```python
from build123d import *

# Parameters (mm, degrees)
SKETCH1_R           = 1.75
BOSS_EXTRUDE1_DEPTH = 3
FILLET1_R           = 0.5


with BuildPart() as part:
    # Sketch1 → Boss-Extrude1 (new body)
    with BuildSketch(Plane.XY):
        with BuildLine():
            Line((-266.5, 139.6), (-179.5, 139.6))
            Line((-179.5, 139.6), (-179.5, 127.873863542))
            ThreePointArc((-179.5, 127.873863542), (-178.955663943, 125.60515051), (-177.441176471, 123.8304144))
            ThreePointArc((-177.441176471, 123.8304144), (-176, 121), (-177.441176471, 118.1695856))
            ThreePointArc((-177.441176471, 118.1695856), (-178.955663943, 116.39484949), (-179.5, 114.126136458))
            Line((-179.5, 114.126136458), (-179.5, 102.4))
            Line((-179.5, 102.4), (-266.5, 102.4))
            Line((-266.5, 102.4), (-266.5, 110))
            Line((-266.5, 110), (-194.5, 110))
            Line((-194.5, 110), (-194.5, 134))
            Line((-194.5, 134), (-266.5, 134))
            Line((-266.5, 134), (-266.5, 139.6))
        make_face()
        with Locations((-179.5, 121)):
            Circle(SKETCH1_R, mode=Mode.SUBTRACT)
    extrude(amount=BOSS_EXTRUDE1_DEPTH)

    # Fillet1
    fillet1_edges = [part.edges().sort_by_distance(p)[0] for p in [
        (-178.955663943, 116.39484949, 0),
        (-179.5, 108.263068229, 0),
        (-179.5, 133.736931771, 3),
        (-223, 102.4, 0),
        (-266.5, 106.2, 0),
        (-230.5, 110, 0),
        (-194.5, 122, 0),
        (-230.5, 134, 0),
        (-266.5, 136.8, 0),
        (-223, 139.6, 0),
        (-179.5, 133.736931771, 0),
        (-178.955663943, 125.60515051, 0),
        (-176, 121, 0),
        (-223, 139.6, 3),
        (-266.5, 136.8, 3),
        (-230.5, 134, 3),
        (-194.5, 122, 3),
        (-181.25, 121, 0),
        (-181.25, 121, 3),
        (-230.5, 110, 3),
        (-266.5, 106.2, 3),
        (-223, 102.4, 3),
        (-179.5, 108.263068229, 3),
        (-178.955663943, 116.39484949, 3),
        (-176, 121, 3),
        (-178.955663943, 125.60515051, 3),
    ]]
    fillet(fillet1_edges, radius=FILLET1_R)


solid = part.part
```
Work out the finished part from the listing and answer in its coordinate system (mm). A direction names the side the tool comes from. Round coordinates to 2 decimals unless told otherwise and drop trailing zeros. Write each loop counter-clockwise with the first axis right and the second up, starting at its lowest first coordinate (ties: lowest second). Pieces come first, ordered by that corner, then holes. Notation, with made-up numbers: (30.5, 1) - (51.5, 1) arc R24 ccw to (51.5, 27) - close; hole circle Ø1 at (47.5, 8.25). An arc over 180 degrees is marked (long way). Return JSON: item names as keys, results as strings. Group by question number.
Q1. The part is cut by section D-D on y = 137. Write down the section's boundary in (x, z), then the cut area to 3 significant figures.
Q2. The part is cut by section B-B on z = 1.2. Write down the section's boundary in (x, y), then the cut area to 3 significant figures.
Q3. The mould has two halves that part along Y. Classify faces 5 (the cylindrical face through (-178.97, 125.63, 1.49)), 6 (the flat face through (-231, 110, 1)), 7 (the flat face through (-211, 109, 3)): released by +Y, released by -Y, zero draft, split by the parting line, or undercut.
Q4. Find the intervals of material crossed by L1, parallel to Y at x = -253.5, z = 0.5; L2, parallel to X at y = 121, z = 1.2; L3, parallel to X at y = 105, z = 1.2, in increasing order.
Q5. Each of these flat-tipped pins is pushed along its axis until it touches: pin 1 Ø1.6 at (y, z) = (118.5, 1) entering from -X; pin 2 Ø12 at (x, y) = (-230, 127) entering from +Z; pin 3 Ø1.6 at (y, z) = (133.5, 1) entering from +X. Where does it stop, or does it pass through?
Q6. The part is cut by section C-C on x = -250. Write down the section's boundary in (y, z), then the cut area to 3 significant figures.
Q7. For faces 1 (the flat face through (-222, 102.4, 1)), 2 (the flat face through (-179.5, 108, 1)), 3 (the flat face through (-194.5, 122, 1)), 4 (the flat face through (-179.5, 134, 1)), determine the directions among +Z, -Z, +X, -X, +Y, -Y from which every point of the face is accessible in a straight line to the end or side of a thin tool.
Q8. The part is cut by section A-A on y = 121. Write down the section's boundary in (x, z), then the cut area to 3 significant figures.
Solved:
{
 "1": {"outline": "(-266.5, 0.5) arc R0.5 ccw to (-266, 0) - (-180, 0) arc R0.5 ccw to (-179.5, 0.5) - (-179.5, 2.5) arc R0.5 ccw to (-180, 3) - (-266, 3) arc R0.5 ccw to (-266.5, 2.5) - close", "area": "261 mm²"},
 "2": {"outline": "(-266.5, 102.4) - (-179.5, 102.4) - (-179.5, 114.13) arc R5 cw to (-177.44, 118.17) arc R3.5 ccw to (-177.44, 123.83) arc R5 cw to (-179.5, 127.87) - (-179.5, 139.6) - (-266.5, 139.6) - (-266.5, 134) - (-194.5, 134) - (-194.5, 110) - (-266.5, 110) - close; hole circle Ø3.5 at (-179.5, 121)", "area": "1,520 mm²"},
 "3": {"face 5": "released by +Y", "face 6": "undercut", "face 7": "zero draft"},
 "4": {"L1": "102.4 to 110, 134 to 139.6", "L2": "-194.5 to -181.25, -177.75 to -176", "L3": "-266.5 to -179.5"},
 "5": {"pin 1": "x = -194.5", "pin 2": "through", "pin 3": "x = -179.5"},
 "6": {"outline": "(102.4, 0.5) arc R0.5 ccw to (102.9, 0) - (109.5, 0) arc R0.5 ccw to (110, 0.5) - (110, 2.5) arc R0.5 ccw to (109.5, 3) - (102.9, 3) arc R0.5 ccw to (102.4, 2.5) - close; (134, 0.5) arc R0.5 ccw to (134.5, 0) - (139.1, 0) arc R0.5 ccw to (139.6, 0.5) - (139.6, 2.5) arc R0.5 ccw to (139.1, 3) - (134.5, 3) arc R0.5 ccw to (134, 2.5) - close", "area": "39.2 mm²"},
 "7": {"face 1": "+Z, -Z, +X, -X, -Y", "face 2": "+Z, -Z, +X, -Y", "face 3": "+Z, -Z, -X", "face 4": "+Z, -Z, +X, +Y"},
 "8": {"outline": "(-194.5, 0.5) arc R0.5 ccw to (-194, 0) - (-181.75, 0) arc R0.5 ccw to (-181.25, 0.5) - (-181.25, 2.5) arc R0.5 ccw to (-181.75, 3) - (-194, 3) arc R0.5 ccw to (-194.5, 2.5) - close; (-177.75, 0.5) arc R0.5 ccw to (-177.25, 0) - (-176.5, 0) arc R0.5 ccw to (-176, 0.5) - (-176, 2.5) arc R0.5 ccw to (-176.5, 3) - (-177.25, 3) arc R0.5 ccw to (-177.75, 2.5) - close", "area": "44.6 mm²"}
}
